Autodesk Inventor part; units mm, degrees
ref_plane "РабПлоскость1" through (10, 0, -2.5) normal (-1, 0, 0) x (0, 0, 1)
ref_plane "YZ Plane" through (0, 0, 0) normal (1, 0, 0) x (0, 1, 0)
ref_plane "XZ Plane" through (0, 0, 0) normal (0, 1, 0) x (-1, 0, 0)
sketch "Эскиз1" plane through (0, 0, 0) normal (0, 1, 0) x (-1, 0, 0)
  circle A0 centre (0, 0) radius 5
  circle A1 centre (0, 0) radius 9
  line L0 (0, 0) -> (0, 2.5)
  line L1 (0, 2.5) -> (20, 2.5)
  line L2 (20, 2.5) -> (20, -2.5)
  line L3 (20, -2.5) -> (0, -2.5)
  point P0 (8.6458, 2.5)
  point P1 (8.6458, -2.5)
  dimension "d0" = 10
  dimension "d1" = 18
  dimension "d2" = 2.5
  dimension "d3" = 20
  dimension "d4" = 5
extrude "Выдавливание1" add sketch "Эскиз1" along normal blind 10 contours A0 L1 A1 L3 | A0 L3 A1 L1 | L1 L2 L3 A1
sketch "Эскиз2" plane through (-20, 0, 2.5) normal (0, 0, 1) x (1, 0, 0)
  line L0 (0, 0) -> (0, 10)
  line L1 (0, 5) -> (20, 5)
  circle A0 centre (20, 5) radius 1.5
  point P0 (20, 0)
  dimension "d7" = 3
extrude "Выдавливание2" cut sketch "Эскиз2" along normal mid plane 35.5
thread "Резьба1"
ref_plane "РабПлоскость1" through (10, 0, -2.5) normal (-1, 0, 0) x (0, 0, 1)
sketch "Эскиз3" plane through (0, 0, 0) normal (0, -1, 0) x (1, 0, 0)
  point P0 (0, 0)
sketch "Эскиз4" plane through (10, 0, -2.5) normal (-1, 0, 0) x (0, 0, 1)
  line L0 (2.5, 0) -> (2.5, 5)
  circle A0 centre (2.5, 5) radius 1.5
  dimension "d13" = 3
hole "Отверстие1" at (10, 5, 0) direction (-1, 0, 0) diameter 2.459 depth 8.8
properties part number "Стопор"
Here's how the part is built. I have some questions about the finished solid (model axes, mm). A direction names the side the tool comes from. Give positions to 0.01 mm unless a question says otherwise; leave off trailing zeros. Write each loop counter-clockwise with the first axis right and the second up, starting at its lowest first coordinate (ties: lowest second). Pieces come first, ordered by that corner, then holes. Notation, with made-up numbers: M -30,73.5 L 29,73.5 A7 cw 29,84.5 Z; hole C -18.5,72.25 d2. An arc over 180 degrees is marked long. Put each result on its own line as item: value. Start each with the question number.
Item 1: Thinking about a two-plate mould opening in X: for faces 1 (the flat face through (-14, 5, 2.5)), 2 (the cylindrical face through (7.02, 4.93, -5.63)), 3 (the cylindrical face through (1.43, 5.45, -6.86)), which applies, +X half, -X half, draft (parallel to the pull), parting line (faces both ways), or undercut?
Item 2: If we section it at B-B, the plane x = 0: Write out the boundary of the cut face in (y, z), then the cut area to 3 significant figures.
Item 3: On a 3-axis mill with a long thin cutter (end or side, diameter ignored), from which of +Z, -Z, +X, -X, +Y, -Y can I reach the whole of each face in a straight line? I mean faces 4 (the flat face through (-14, 5, -2.5)), 5 (the cylindrical face through (6.89, 6.2, 0.27)), 6 (the cylindrical face through (-4.619, 4.93, 1.915)). Say none if no direction works.
Item 4: If we section it at A-A, the plane z = 0: Write out the boundary of the cut face in (x, y), then the cut area to 3 significant figures.
Item 5: If we section it at C-C, the plane y = 5: Write out the boundary of the cut face in (x, z), then the cut area to 3 significant figures.
Item 6: I need wall thicknesses on L1, parallel to X at y = 8.25, z = 0.25; L2, parallel to Y at x = 6.2, z = 0; L3, parallel to X at y = 4, z = -6.5. Which ranges of each line are inside material? Lowest first, please. Write a range as from..to.
Item 7: If we section it at D-D, the plane y = 8.5: Write out the boundary of the cut face in (x, z), then the cut area to 3 significant figures.
Item 8: Will these pins go through, and if not, where does the flat tip stop? pin 1 (4 mm diameter, centred on y = 5, z = 0, fed in from +X); pin 2 (2 mm diameter, centred on x = 1.5, y = 2.5, fed in from +Z); pin 3 (5 mm diameter, centred on x = -13.5, y = 6, fed in from +Z); pin 4 (5 mm diameter, centred on x = -17, y = 4, fed in from -Z).
Values:
1. face 1: draft
1. face 2: parting line
1. face 3: undercut
2. outline: M 0,-9 L 3.5,-9 L 3.5,-5 L 0,-5 Z; M 0,5 L 3.5,5 L 3.5,9 L 0,9 Z; M 6.5,-9 L 10,-9 L 10,-5 L 6.5,-5 Z; M 6.5,5 L 10,5 L 10,9 L 6.5,9 Z
2. area: 56.0 mm²
3. face 4: -Z, -X, +Y, -Y
3. face 5: +X
3. face 6: +Y, -Y
4. outline: M -20,0 L -5,0 L -5,10 L -20,10 Z; M 5,0 L 9,0 L 9,3.77 L 5,3.77 Z; M 5,6.23 L 9,6.23 L 9,10 L 5,10 Z
4. area: 180 mm²
5. outline: M -20,-2.5 L -8.65,-2.5 A9 ccw -1.5,-8.87 L -1.5,-4.77 A5 cw -1.5,4.77 L -1.5,8.87 A9 ccw -8.65,2.5 L -20,2.5 Z; M 1.5,-8.87 A9 ccw 8.92,-1.23 L 4.85,-1.23 A5 cw 1.5,-4.77 Z; M 1.5,4.77 A5 cw 4.85,1.23 L 8.92,1.23 A9 ccw 1.5,8.87 Z
5. area: 197 mm²
6. L1: -20..-4.99, 4.99..9
6. L2: 0..3.77, 6.23..10
6. L3: -6.22..-1.12, 1.12..6.22
7. outline: M -20,-2.5 L -8.65,-2.5 A9 ccw long -8.65,2.5 L -20,2.5 Z; hole C 0,0 d10
7. area: 232 mm²
8. pin 1: x = 9
8. pin 2: z = 8.99
8. pin 3: z = 2.5
8. pin 4: z = -2.5
